The model under review builds one solid part; all positions refer to its coordinate system, in mm. Face numbers are marked on the shaded views. A direction names the side the tool comes from. Coordinates: 2 decimals unless noted, no trailing zeros. Order: outer loops, then holes, each group sorted by start corner. A loop starts at its lowest first (then second) coordinate and runs counter-clockwise, first axis right, second up. Notation, with made-up numbers: M 57.25,60.5 L 75.25,60.5 A9 cw 75.25,67.5 Z; hole C -10.75,20 d5. An arc over 180 degrees is marked long. One line per item, written item: value.
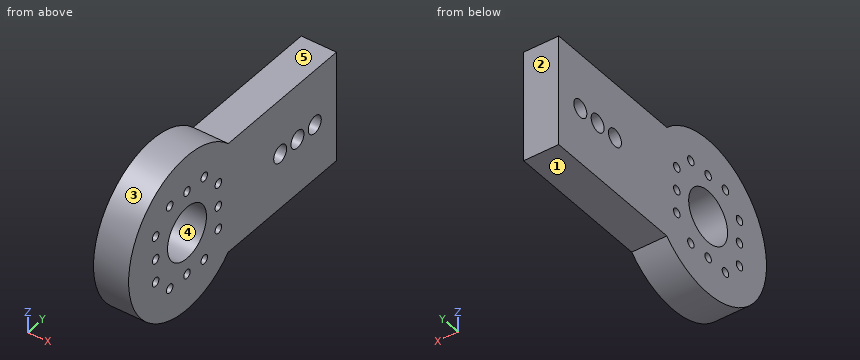
```python
from build123d import *

# Parameters (mm, degrees)
SKETCH1_R           = 4.5
SKETCH1_R_2         = 0.75
SKETCH1_R_3         = 1.5
SKETCH1_R_4         = 1.498254454
BOSS_EXTRUDE1_DEPTH = 6


with BuildPart() as part:
    # Sketch1 → Boss-Extrude1 (new body)
    with BuildSketch(Plane(origin=(0, 0, 0), x_dir=(0, 0, -1), z_dir=(1, 0, 0))):
        with BuildLine():
            Line((-9.542574057, 9.549307848), (-9.542574057, 34.549307848))
            Line((-9.542574057, 34.549307848), (9.542574057, 34.549307848))
            Line((9.542574057, 34.549307848), (9.542574057, 9.549307848))
            ThreePointArc((9.542574057, 9.549307848), (0, -13.5), (-9.542574057, 9.549307848))
        make_face()
        Circle(SKETCH1_R, mode=Mode.SUBTRACT)
        with Locations((0, 7.25)):
            Circle(SKETCH1_R_2, mode=Mode.SUBTRACT)
        with Locations((4, 7.25)):
            Circle(SKETCH1_R_2, mode=Mode.SUBTRACT)
        with Locations((-4, 7.25)):
            Circle(SKETCH1_R_2, mode=Mode.SUBTRACT)
        with Locations(Location((4, -7.25, 0), (0, 0, 180))):
            Circle(SKETCH1_R_2, mode=Mode.SUBTRACT)
        with Locations(Location((0, -7.25, 0), (0, 0, 180))):
            Circle(SKETCH1_R_2, mode=Mode.SUBTRACT)
        with Locations(Location((-4, -7.25, 0), (0, 0, 180))):
            Circle(SKETCH1_R_2, mode=Mode.SUBTRACT)
        with Locations((7.25, -4)):
            Circle(SKETCH1_R_2, mode=Mode.SUBTRACT)
        with Locations((7.25, 0)):
            Circle(SKETCH1_R_2, mode=Mode.SUBTRACT)
        with Locations((7.25, 4)):
            Circle(SKETCH1_R_2, mode=Mode.SUBTRACT)
        with Locations((-7.25, 4)):
            Circle(SKETCH1_R_2, mode=Mode.SUBTRACT)
        with Locations((-7.25, 0)):
            Circle(SKETCH1_R_2, mode=Mode.SUBTRACT)
        with Locations((-7.25, -4)):
            Circle(SKETCH1_R_2, mode=Mode.SUBTRACT)
        with Locations((0, 29.549307848)):
            Circle(SKETCH1_R_3, mode=Mode.SUBTRACT)
        with Locations((0, 25.549307848)):
            Circle(SKETCH1_R_3, mode=Mode.SUBTRACT)
        with Locations((0, 21.549307848)):
            Circle(SKETCH1_R_4, mode=Mode.SUBTRACT)
    extrude(amount=BOSS_EXTRUDE1_DEPTH)


solid = part.part
```
(1) Mouldability with a two-part tool opening along Y and no side actions: class the marked faces 3, 4 and 5 as +Y half, -Y half, draft (parallel to the pull), parting line (faces both ways), or undercut.
Geometry results:
face 3: parting line
face 4: undercut
face 5: draft
(2) We need section C-C, the plane x = 2.35. Count the separate pieces of the cut face and the enclosed holes in it, plus the area to 3 significant figures.
Geometry results:
separate pieces: 1
enclosed holes: 16
area: 892 mm2
(3) Insertion check: pin 1 Ø1.5 at (x, y) = (3, 12) entering from +Z; pin 2 Ø1 at (x, z) = (1, 10.5) entering from -Y. Each pin has a flat end and moves straight along its axis. Give the tip position at first contact, or say it passes through.
Geometry results:
pin 1: stops at z = 9.54
pin 2: stops at y = -9.07
(4) We need section D-D, the plane z = -7.25. State the section outline as (x, y) points, plus the area to 3 significant figures.
Geometry results:
outline: M 0,-11.39 L 6,-11.39 L 6,-4.75 L 0,-4.75 Z; M 0,-3.25 L 6,-3.25 L 6,-0.75 L 0,-0.75 Z; M 0,0.75 L 6,0.75 L 6,3.25 L 0,3.25 Z; M 0,4.75 L 6,4.75 L 6,34.55 L 0,34.55 Z
area: 249 mm2
(5) For L1, parallel to Y at x = 2.7, z = 7.5; L2, parallel to Y at x = 1.2, z = -7.25; L3, parallel to Z at x = 1.25, y = 7.5, list the stretches that pass through material, from the lowest coordinate up.
Geometry results:
L1: y = -11.22 to -4.71, -3.29 to -0.71, 0.71 to 3.29, 4.71 to 34.55
L2: y = -11.39 to -4.75, -3.25 to -0.75, 0.75 to 3.25, 4.75 to 34.55
L3: z = -11.22 to -4.71, -3.29 to -0.71, 0.71 to 3.29, 4.71 to 11.22
(6) We need section A-A, the plane z = 0. State the section outline as (x, y) points.
Geometry results:
outline: M 0,-13.5 L 6,-13.5 L 6,-8 L 0,-8 Z; M 0,-6.5 L 6,-6.5 L 6,-4.5 L 0,-4.5 Z; M 0,4.5 L 6,4.5 L 6,6.5 L 0,6.5 Z; M 0,8 L 6,8 L 6,20.05 L 0,20.05 Z; M 0,23.05 L 6,23.05 L 6,24.05 L 0,24.05 Z; M 0,27.05 L 6,27.05 L 6,28.05 L 0,28.05 Z; M 0,31.05 L 6,31.05 L 6,34.55 L 0,34.55 Z
(7) Tool access review of the marked faces 1 and 2: name each direction out of +Z, -Z, +X, -X, +Y, -Y from which nothing blocks a thin tool from reaching the whole face with its end or side.
Geometry results:
face 1: -Z, +X, -X, +Y
face 2: +Z, -Z, +X, -X, +Y
(8) We need section B-B, the plane y = -4. State the section outline as (x, z) points, plus the area to 3 significant figures.
Geometry results:
outline: M 0,-12.89 L 6,-12.89 L 6,-8 L 0,-8 Z; M 0,-6.5 L 6,-6.5 L 6,-2.06 L 0,-2.06 Z; M 0,2.06 L 6,2.06 L 6,6.5 L 0,6.5 Z; M 0,8 L 6,8 L 6,12.89 L 0,12.89 Z
area: 112 mm2
